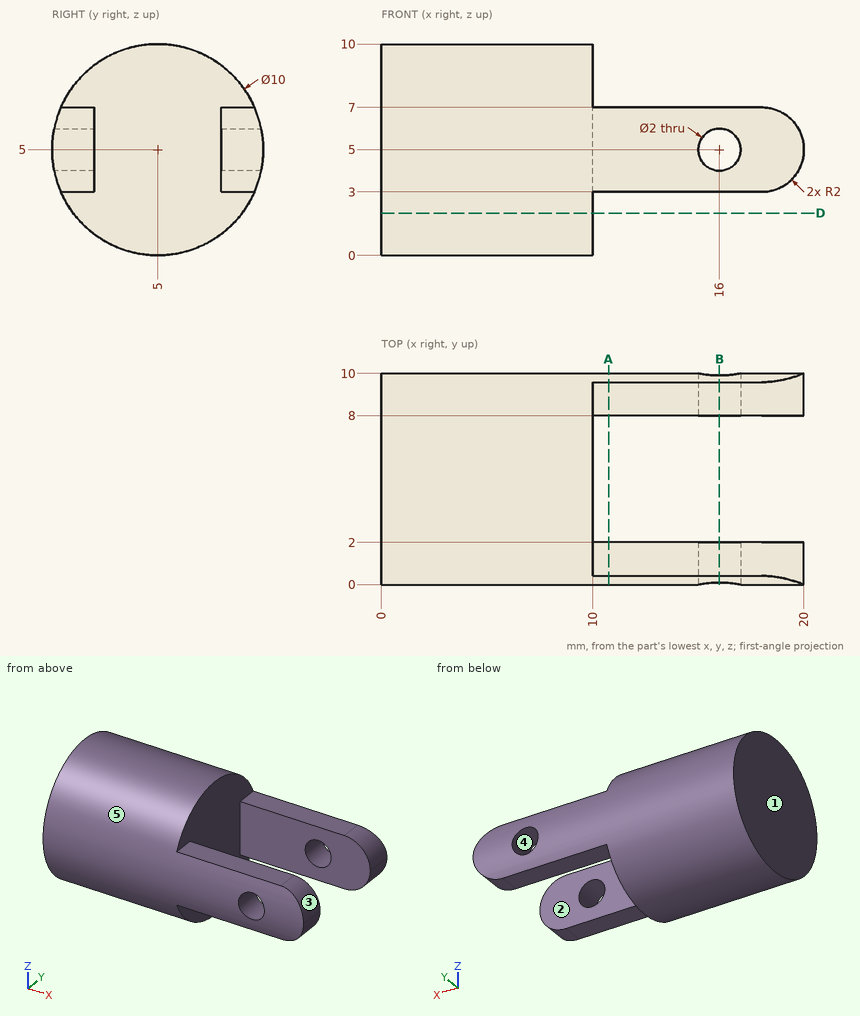
Geometry: see drawing. Coordinates: mm, zero at the bounding-box minimum. A direction names the side the tool comes from. Round coordinates to 2 decimals unless told otherwise and drop trailing zeros. Loops run counter-clockwise (first coordinate to the right, second up) from the corner with the lowest first, then second, coordinate; pieces in that order, holes last. Notation, with made-up numbers: (5, -11.5) -> (59, -11.5) arc R7 ccw to (59, -5.5) -> close; hole circle Ø2 at (66.5, 11). An arc over 180 degrees is marked (long way). Use one line per item in the form item = value. Start each with the question number.
Item 1: Section query A-A on x = 10.75. Return the cut outline in (y, z).
Item 2: Contact query for flat-ended pins moving along their axis: pin 1 Ø1.2 at (x, z) = (15, 6) entering from -Y; pin 2 Ø1.7 at (x, y) = (14, 1) entering from +Z; pin 3 Ø0.5 at (x, y) = (13, 1) entering from -Z. Output: stop coordinate, or through.
Item 3: Mould query, pull axis Z, two halves, no side actions, for the marked faces 3, 4 and 5. Classes: pulls with the +Z half, pulls with the -Z half, needs draft (parallel to the pull), parting line crosses it, or undercut.
Item 4: Section query D-D on z = 2. Return the cut outline in (x, y), then the cut area to 3 significant figures.
Item 5: Set-up query: the marked faces 1 and 2. Return all of +Z, -Z, +X, -X, +Y, -Y with unobstructed straight access to the full face (end or side cutting, diameter ignored); none if empty.
Item 6: Section query B-B on x = 16. Return the cut outline in (y, z), then the cut area to 3 significant figures.
Item 7: Material intervals for L1, parallel to X at y = 8.95, z = 5; L2, parallel to X at y = 1.75, z = 2.25; L3, parallel to Z at x = 9, y = 3, sorted ascending. Write a range as from..to.
Ans:
q1.outline = (0.42, 3) -> (2, 3) -> (2, 7) -> (0.42, 7) arc R5 ccw to start; (8, 3) -> (9.58, 3) arc R5 ccw to (9.58, 7) -> (8, 7) -> close
q2.pin_1 = 0.02
q2.pin_2 = 7
q2.pin_3 = 3
q3.face_3 = pulls with the +Z half
q3.face_4 = undercut
q3.face_5 = parting line crosses it
q4.outline = (0, 1) -> (10, 1) -> (10, 9) -> (0, 9) -> close
q4.area = 80.0 mm^2
q5.face_1 = +Z, -Z, -X, +Y, -Y
q5.face_2 = +Z, -Z, +X
q6.outline = (0.1, 4) arc R5 ccw to (0.42, 3) -> (2, 3) -> (2, 4) -> close; (0.1, 6) -> (2, 6) -> (2, 7) -> (0.42, 7) arc R5 ccw to start; (8, 3) -> (9.58, 3) arc R5 ccw to (9.9, 4) -> (8, 4) -> close; (8, 6) -> (9.9, 6) arc R5 ccw to (9.58, 7) -> (8, 7) -> close
q6.area = 7.04 mm^2
q7.L1 = 0..15, 17..20
q7.L2 = 0..10
q7.L3 = 0.42..9.58
